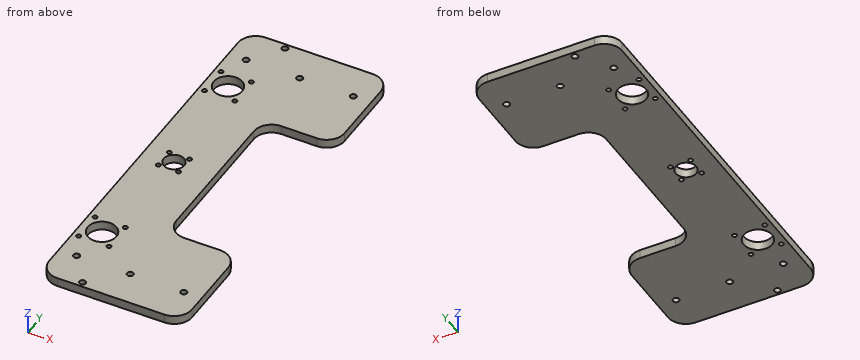
from build123d import *

# Parameters (mm, degrees)
PAD_DEPTH            = 5
SKETCH002_R          = 8
SKETCH002_R_2        = 1.25
POCKET_DEPTH         = 458.912756
POCKET_DEPTH_BACK    = 463.912756
SKETCH004_R          = 1.75
POCKET001_DEPTH      = 458.912756
POCKET001_DEPTH_BACK = 463.912756
SKETCH003_R          = 1.75
POCKET002_DEPTH      = 458.912756
POCKET002_DEPTH_BACK = 463.912756
SKETCH005_R          = 5.75
SKETCH005_R_2        = 1.25
POCKET003_DEPTH      = 0.001
POCKET003_DEPTH_BACK = 5.001


with BuildPart() as part:
    # Sketch001 → Pad (new body)
    with BuildSketch(Plane.XY):
        with BuildLine():
            Line((88, -97.5), (88, -60))
            ThreePointArc((88, -60), (85.071068, -52.928932), (78, -50))
            Line((58, -50), (78, -50))
            ThreePointArc((48, -40), (50.928932, -47.071068), (58, -50))
            Line((48, -40), (48, 40))
            ThreePointArc((58, 50), (50.928932, 47.071068), (48, 40))
            Line((58, 50), (78, 50))
            ThreePointArc((78, 50), (85.071068, 52.928932), (88, 60))
            Line((88, 97.5), (88, 60))
            ThreePointArc((88, 97.5), (85.071068, 104.571068), (78, 107.5))
            Line((18, 107.5), (78, 107.5))
            ThreePointArc((18, 107.5), (10.928932, 104.571068), (8, 97.5))
            Line((8, 97.5), (8, -97.5))
            ThreePointArc((8, -97.5), (10.928932, -104.571068), (18, -107.5))
            Line((18, -107.5), (78, -107.5))
            ThreePointArc((78, -107.5), (85.071068, -104.571068), (88, -97.5))
        make_face()
    extrude(amount=PAD_DEPTH)

    # Sketch002 → Pocket (cut, two sides)
    with BuildSketch(Plane.XY) as pocket_sk:
        with Locations((20, -65)):
            Circle(SKETCH002_R)
        with Locations((11.514719, -56.514719)):
            Circle(SKETCH002_R_2)
        with Locations((11.514719, -73.485281)):
            Circle(SKETCH002_R_2)
        with Locations((28.485281, -73.485281)):
            Circle(SKETCH002_R_2)
        with Locations((28.485281, -56.514719)):
            Circle(SKETCH002_R_2)
    pocket = extrude(amount=-POCKET_DEPTH, mode=Mode.SUBTRACT) + extrude(pocket_sk.sketch, amount=POCKET_DEPTH_BACK, mode=Mode.SUBTRACT)

    # Mirrored: Pocket across Sketch002 Axis6
    add(pocket.mirror(Plane(origin=(-25, 0, 0), x_dir=(0, 0, 1), z_dir=(0, 1, 0))), mode=Mode.SUBTRACT)

    # Sketch004 → Pocket001 (cut, two sides)
    with BuildSketch(Plane.XY) as pocket001_sk:
        with Locations((78, -87.5)):
            Circle(SKETCH004_R)
        with Locations((48, -87.5)):
            Circle(SKETCH004_R)
        with Locations((18, -87.5)):
            Circle(SKETCH004_R)
    pocket001 = extrude(amount=-POCKET001_DEPTH, mode=Mode.SUBTRACT) + extrude(pocket001_sk.sketch, amount=POCKET001_DEPTH_BACK, mode=Mode.SUBTRACT)

    # Mirrored001: Pocket001 across Sketch004 Axis0
    add(pocket001.mirror(Plane(origin=(-25, 0, 0), x_dir=(0, 0, 1), z_dir=(0, 1, 0))), mode=Mode.SUBTRACT)

    # Sketch003 → Pocket002 (cut, two sides)
    with BuildSketch(Plane.XY) as pocket002_sk:
        with Locations((30.5, -104.5)):
            Circle(SKETCH003_R)
    pocket002 = extrude(amount=-POCKET002_DEPTH, mode=Mode.SUBTRACT) + extrude(pocket002_sk.sketch, amount=POCKET002_DEPTH_BACK, mode=Mode.SUBTRACT)

    # Mirrored002: Pocket002 across Sketch003 Axis0
    add(pocket002.mirror(Plane(origin=(-25, 0, 0), x_dir=(0, 0, 1), z_dir=(0, 1, 0))), mode=Mode.SUBTRACT)

    # Sketch005 → Pocket003 (cut, two sides)
    with BuildSketch(Plane.XY) as pocket003_sk:
        with Locations((25, 0)):
            Circle(SKETCH005_R)
        with Locations((30.656854, -5.656854)):
            Circle(SKETCH005_R_2)
        with Locations((30.656854, 5.656854)):
            Circle(SKETCH005_R_2)
        with Locations((19.343146, 5.656854)):
            Circle(SKETCH005_R_2)
        with Locations((19.343146, -5.656854)):
            Circle(SKETCH005_R_2)
    extrude(amount=-POCKET003_DEPTH, mode=Mode.SUBTRACT)
    extrude(pocket003_sk.sketch, amount=POCKET003_DEPTH_BACK, mode=Mode.SUBTRACT)


solid = part.part
Geometry check sheet. Reference: the model listing, model coordinates, mm. Coordinates: 2 decimals unless noted, no trailing zeros. Order: outer loops, then holes, each group sorted by start corner. A loop starts at its lowest first (then second) coordinate and runs counter-clockwise, first axis right, second up. Notation, with made-up numbers: (79, 5.5) - (116, 5.5) arc R27 cw to (116, 37.5) - close; hole circle Ø4 at (5, 50). An arc over 180 degrees is marked (long way). One line per item, written item: value.
(1) Sectioned sample at A-A (y = 0). Enter the section's corners in (x, z), and give its area (4 significant figures).
Data:
outline: (8, 0) - (19.25, 0) - (19.25, 5) - (8, 5) - close; (30.75, 0) - (48, 0) - (48, 5) - (30.75, 5) - close
area: 142.5 mm^2
(2) Depth check by flat-ended pin: pin 1 Ø3 at (x, y) = (24, -33) entering from -Z. Enter the tip coordinate at first touch or a pass-through.
Data:
pin 1: stops at z = 0
(3) Sectioned sample at C-C (z = 1.75). Count the separate pieces of the cut face and the enclosed holes in it, and give its area (3 significant figures).
Data:
separate pieces: 1
enclosed holes: 23
area: 12,500 mm^2
(4) Thickness scan on probe 1 along Y at (x, z) = (78, 3.7); probe 2 along X at (y, z) = (87.5, 1.45); probe 3 along Y at (x, z) = (59, 1.6). Record the ranges inside material, lowest first. Write a range as from..to.
Data:
probe 1: y = -107.5..-89.25, -85.75..-50, 50..85.75, 89.25..107.5
probe 2: x = 8..16.25, 19.75..46.25, 49.75..76.25, 79.75..88
probe 3: y = -107.5..-50, 50..107.5
(5) Sectioned sample at B-B (x = 64.5). Enter the section's corners in (y, z).
Data:
outline: (-107.5, 0) - (-50, 0) - (-50, 5) - (-107.5, 5) - close; (50, 0) - (107.5, 0) - (107.5, 5) - (50, 5) - close
